For this review, take the finished solid that the model builds, in its own axes (mm). A direction names the side the tool comes from. Coordinates: 2 decimals unless noted, no trailing zeros. Order: outer loops, then holes, each group sorted by start corner. A loop starts at its lowest first (then second) coordinate and runs counter-clockwise, first axis right, second up.
from build123d import *

# Parameters (mm, degrees)
F0_R     = 15.875
F1_DEPTH = 44.45
F2_DEPTH = 25.4
F0_R_2   = 9.525
F3_DEPTH = 15.24


with BuildPart() as f1:
    # F0 (on Front) → F1 (new body)
    with BuildSketch(Plane.XZ):
        with BuildLine():
            ThreePointArc((28.575, 0), (22.018516, 18.21306), (5.357812, 28.068211))
            ThreePointArc((5.357812, 28.068211), (-28.575, 0), (5.357812, -28.068211))
            ThreePointArc((5.357812, -28.068211), (22.018516, -18.21306), (28.575, 0))
        make_face()
        Circle(F0_R, mode=Mode.SUBTRACT)
    extrude(amount=F1_DEPTH)

    # F0 (on Front) → F2 (join)
    with BuildSketch(Plane.XZ):
        with BuildLine():
            ThreePointArc((54.371875, -18.712141), (31.75, 0), (54.371875, 18.712141))
            Line((54.371875, 18.712141), (5.357812, 28.068211))
            ThreePointArc((5.357812, 28.068211), (22.018516, 18.21306), (28.575, 0))
            ThreePointArc((28.575, 0), (22.018516, -18.21306), (5.357812, -28.068211))
            Line((5.357812, -28.068211), (54.371875, -18.712141))
        make_face()
    extrude(amount=F2_DEPTH)

    # F0 (on Front) → F3 (join)
    with BuildSketch(Plane.XZ):
        with BuildLine():
            ThreePointArc((54.371875, -18.712141), (65.479011, -12.14204), (69.85, 0))
            ThreePointArc((69.85, 0), (65.479011, 12.14204), (54.371875, 18.712141))
            ThreePointArc((54.371875, 18.712141), (31.75, 0), (54.371875, -18.712141))
        make_face()
        with Locations((50.8, 0)):
            Circle(F0_R_2, mode=Mode.SUBTRACT)
    extrude(amount=F3_DEPTH)


solid = f1.part
1. Take a section at C-C, the plane y = -4. Give the boundary of the cut face in (x, z) (3 decimals), plus the area to 3 significant figures.
Answer below:
outline: (5.358, -28.068) - (54.372, -18.712) arc R19.05 ccw to (54.372, 18.712) - (5.358, 28.068) arc R28.575 ccw (long way) to start; hole circle Ø31.75 at (0, 0); hole circle Ø19.05 at (50.8, 0)
area: 3,240 mm2
2. Clearance check with flat-ended pins moving along their axes: pin 1 Ø2 at (y, z) = (-28.5, -17.5) entering from +X; pin 2 Ø2 at (y, z) = (-24, -15) entering from -X; pin 3 Ø1 at (x, z) = (48.5, 15.5) entering from -Y; pin 4 Ø12 at (x, z) = (-1, 15) entering from -Y. State where each tip first meets the part, or that it passes through.
Answer below:
pin 1: stops at x = 23.33
pin 2: stops at x = -24.91
pin 3: stops at y = -15.24
pin 4: stops at y = -44.45
3. Machinability: for faces 5 (the face through (31.756, -20.249, -0.469)), 6 (the face through (20, 0, 0)), which of the approach directions +Z, -Z, +X, -X, +Y, -Y give a long, thin tool a straight path to every point of the face, cutting with its end or side? Answer none if there is none.
Answer below:
face 5: -Y
face 6: +Z, -Z, +X, -X, +Y
4. Take a section at A-A, the plane x = 0. Give the boundary of the cut face in (y, z) (3 decimals), plus the area to 3 significant figures.
Answer below:
outline: (-44.45, -28.575) - (0, -28.575) - (0, -15.875) - (-44.45, -15.875) - close; (-44.45, 15.875) - (0, 15.875) - (0, 28.575) - (-44.45, 28.575) - close
area: 1,130 mm2
5. Take a section at B-B, the plane z = 2. Give the boundary of the cut face in (x, y).
Answer below:
outline: (-28.5, -44.45) - (-15.75, -44.45) - (-15.75, 0) - (-28.5, 0) - close; (15.75, -44.45) - (28.5, -44.45) - (28.5, -25.4) - (31.86, -25.4) - (31.86, -15.24) - (41.49, -15.24) - (41.49, 0) - (15.75, 0) - close; (60.11, -15.24) - (69.74, -15.24) - (69.74, 0) - (60.11, 0) - close
6. To check wall thickness, follow L1, parallel to Z at x = 0, y = -19 (3 decimals); L2, parallel to Y at x = 57.5, z = -17; L3, parallel to X at y = -8.5, z = -7. State the ranges of each line that lie inside material, in increasing order.
Answer below:
L1: z = -28.575 to -15.875, 15.875 to 28.575
L2: y = -15.24 to 0
L3: x = -27.7 to -14.25, 14.25 to 44.34, 57.26 to 68.52
7. Take a section at D-D, the plane y = -27.5. Give the boundary of the cut face in (x, z) (3 decimals), plus the area to 3 significant figures.
Answer below:
outline: (5.358, -28.068) arc R28.575 ccw to (28.575, 0) arc R28.575 ccw to (5.358, 28.068) arc R28.575 ccw (long way) to start; hole circle Ø31.75 at (0, 0)
area: 1,770 mm2
8. The part is to be moulded in two halves that separate along Z. For faces 1 (the face through (55, -15.24, 9)), 2 (the face through (30, -25.4, 2)), 3 (the face through (29.522, -12.522, -23.456)), 4 (the face through (59.6, -7.51, -3.65)), say which applies: +Z half, -Z half, draft (parallel to the pull), parting line (faces both ways), or undercut.
Answer below:
face 1: undercut
face 2: draft
face 3: -Z half
face 4: undercut
